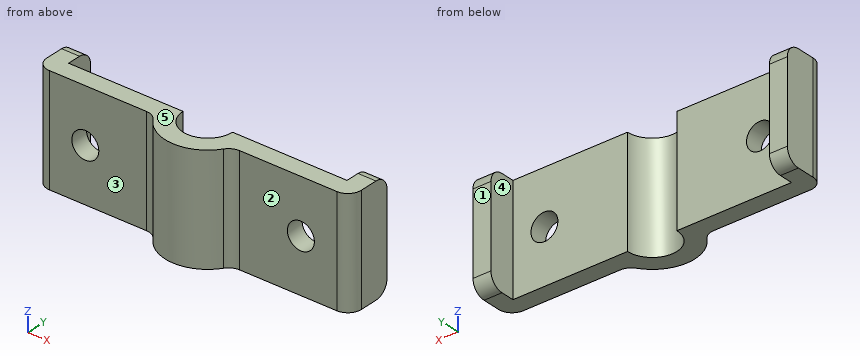
```python
from build123d import *

# Parameters (mm, degrees)
F1_DEPTH = 76.2
F2_R     = 9.525
F5_DEPTH = 25.4


with BuildPart() as f1:
    # F0 (on Top) → F1 (new body)
    with BuildSketch(Plane.XY):
        with BuildLine():
            Line((0, -31.75), (0, 0))
            Line((0, 0), (-12.7, 0))
            Line((-12.7, 0), (-12.7, -19.05))
            Line((-12.7, -19.05), (-80.9625, -19.05))
            ThreePointArc((-80.9625, -19.05), (-81.671846117, -25.552932615), (-83.7665203959, -31.75))
            Line((-83.7665203959, -31.75), (0, -31.75))
        make_face()
        with BuildLine():
            Line((-222.25, -31.75), (-138.4834796041, -31.75))
            ThreePointArc((-138.4834796041, -31.75), (-140.578153883, -25.552932615), (-141.2875, -19.05))
            Line((-141.2875, -19.05), (-209.55, -19.05))
            Line((-209.55, -19.05), (-209.55, 0))
            Line((-209.55, 0), (-222.25, 0))
            Line((-222.25, 0), (-222.25, -31.75))
        make_face()
        with BuildLine():
            ThreePointArc((-138.4834796041, -31.75), (-111.125, -49.2125), (-83.7665203959, -31.75))
            Line((-83.7665203959, -31.75), (-99.139637834, -31.75))
            ThreePointArc((-99.139637834, -31.75), (-111.125, -36.5125), (-123.110362166, -31.75))
            Line((-123.110362166, -31.75), (-138.4834796041, -31.75))
        make_face()
        with BuildLine():
            ThreePointArc((-141.2875, -19.05), (-140.578153883, -25.552932615), (-138.4834796041, -31.75))
            Line((-138.4834796041, -31.75), (-123.110362166, -31.75))
            ThreePointArc((-123.110362166, -31.75), (-127.1598572347, -25.9653640333), (-128.5875, -19.05))
            Line((-128.5875, -19.05), (-141.2875, -19.05))
        make_face()
        with BuildLine():
            Line((-99.139637834, -31.75), (-83.7665203959, -31.75))
            ThreePointArc((-83.7665203959, -31.75), (-81.671846117, -25.552932615), (-80.9625, -19.05))
            Line((-80.9625, -19.05), (-93.6625, -19.05))
            ThreePointArc((-93.6625, -19.05), (-95.0901427653, -25.9653640333), (-99.139637834, -31.75))
        make_face()
    extrude(amount=F1_DEPTH)

    # F2
    f2_edges = [f1.edges().sort_by_distance(p)[0] for p in [
        (-6.35, 0, 0),
        (-6.35, 0, 76.2),
        (-215.9, 0, 76.2),
        (-215.9, 0, 0),
        (0, -31.75, 38.1),
        (-222.25, -31.75, 38.1),
        (-83.76652, -31.75, 38.1),
        (-138.48348, -31.75, 38.1),
    ]]
    fillet(f2_edges, radius=F2_R)

    # F4 (on face) + F3 (on face) → F5 (cut)
    with BuildSketch(Plane.XZ.offset(31.75)):
        with BuildLine():
            ThreePointArc((-25.4121996562, 38.1), (-28.2020075654, 44.8351920908), (-34.9371996562, 47.625))
            Line((-34.9371996562, 47.625), (-34.9371996562, 38.1))
            Line((-34.9371996562, 38.1), (-34.9371996562, 28.575))
            ThreePointArc((-34.9371996562, 28.575), (-28.2020075654, 31.3648079092), (-25.4121996562, 38.1))
        make_face()
        with BuildLine():
            Line((-34.9371996562, 38.1), (-34.9371996562, 47.625))
            ThreePointArc((-34.9371996562, 47.625), (-44.4621996562, 38.1), (-34.9371996562, 28.575))
            Line((-34.9371996562, 28.575), (-34.9371996562, 38.1))
        make_face()
    with BuildSketch(Plane.XZ.offset(31.75)):
        with BuildLine():
            ThreePointArc((-177.7878003438, 38.1), (-180.577608253, 44.8351920908), (-187.3128003438, 47.625))
            Line((-187.3128003438, 47.625), (-187.3128003438, 38.1))
            Line((-187.3128003438, 38.1), (-187.3128003438, 28.575))
            ThreePointArc((-187.3128003438, 28.575), (-180.577608253, 31.3648079092), (-177.7878003438, 38.1))
        make_face()
        with BuildLine():
            Line((-187.3128003438, 38.1), (-187.3128003438, 47.625))
            ThreePointArc((-187.3128003438, 47.625), (-196.8378003438, 38.1), (-187.3128003438, 28.575))
            Line((-187.3128003438, 28.575), (-187.3128003438, 38.1))
        make_face()
    extrude(amount=-F5_DEPTH, mode=Mode.SUBTRACT)


solid = f1.part
```
Input: part model. Units: mm. Frame: model coordinates. Face numbers are marked on the shaded views. A direction names the side the tool comes from. Coordinates: 2 decimals unless noted, no trailing zeros. Write each loop counter-clockwise with the first axis right and the second up, starting at its lowest first coordinate (ties: lowest second). Pieces come first, ordered by that corner, then holes. Notation, with made-up numbers: M -19.5,25 L -1.5,25 A23 ccw -1.5,43 Z; hole C 88,80.5 d7. An arc over 180 degrees is marked long. Use one line per item in the form item = value.
Q1. Material intervals for probe 1 along X at (y, z) = (-12, 27.5); probe 2 along X at (y, z) = (-24, 38); probe 3 along X at (y, z) = (-25.5, 38.1), sorted ascending. Write a range as from..to.
Answer below:
probe_1 = -222.25..-209.55, -12.7..0
probe_2 = -222.08..-196.84, -177.79..-127.87, -94.38..-44.46, -25.41..-0.17
probe_3 = -221.67..-196.84, -177.79..-127.35, -94.9..-44.46, -25.41..-0.58
Q2. First-contact query: pin 1 (3 mm diameter, centred on x = -56, z = 50.5, fed in from +Y); pin 2 (6 mm diameter, centred on x = -28.5, y = -25.5, fed in from -Z); pin 3 (8 mm diameter, centred on x = -83.5, z = 45.5, fed in from -Y); pin 4 (25 mm diameter, centred on x = -34.94, z = 38.1, fed in from -Y). Flat tips, straight axial feed; report the tip coordinate or a pass-through.
Answer below:
pin_1 = -19.05
pin_2 = 0
pin_3 = -37.8
pin_4 = -31.75
Q3. Section B-B (y = -14). Return loops of the section in (x, z).
Answer below:
outline = M -222.25,0 L -209.55,0 L -209.55,76.2 L -222.25,76.2 Z; M -12.7,0 L 0,0 L 0,76.2 L -12.7,76.2 Z
Q4. Section D-D (x = -54). Return loops of the section in (y, z).
Answer below:
outline = M -31.75,0 L -19.05,0 L -19.05,76.2 L -31.75,76.2 Z
Q5. Set-up query: the marked faces 1, 2, 3, 4 and 5. Return all of +Z, -Z, +X, -X, +Y, -Y with unobstructed straight access to the full face (end or side cutting, diameter ignored); none if empty.
Answer below:
face_1 = +Z, -Z, +X, -X, +Y
face_2 = +Z, -Z, +X, -Y
face_3 = +Z, -Z, -X, -Y
face_4 = +Z, -Z, +Y
face_5 = +Z, +X, -X, +Y, -Y
Q6. Section A-A (z = 38.1). Count the separate pieces of the cut face and the enclosed holes in it, plus the area to 3 significant figures.
Answer below:
separate_pieces = 3
enclosed_holes = 0
area = 3,000 mm²
